```python
from build123d import *

# Parameters (mm, degrees)
SALIENTE_EXTRUIR1_DEPTH      = 22
CROQUIS2_W                   = 43.142135624
CROQUIS2_H                   = 44
SALIENTE_EXTRUIR2_DEPTH      = 8
CROQUIS3_W                   = 33.76116098
CROQUIS3_H                   = 8
CORTAR_EXTRUIR1_DEPTH        = 49.74935897
CROQUIS4_R                   = 11
SALIENTE_EXTRUIR4_DEPTH      = 2
CROQUIS7_R                   = 16
CROQUIS7_R_2                 = 2.6
SALIENTE_EXTRUIR5_DEPTH      = 2
CROQUIS6_W                   = 28
CROQUIS6_H                   = 12
CORTAR_EXTRUIR3_DEPTH        = 13
SALIENTE_EXTRUIR6_DEPTH      = 12
SALIENTE_EXTRUIR6_DEPTH_BACK = 3.8
CROQUIS8_W                   = 12
CROQUIS8_H                   = 12
CROQUIS8_R                   = 1.6
CROQUIS9_W                   = 2.5
CROQUIS9_H                   = 5.6
CORTAR_EXTRUIR4_DEPTH        = 10
CROQUIS11_W                  = 43.142135624
CROQUIS11_H                  = 46
SALIENTE_EXTRUIR8_DEPTH      = 30
CROQUIS12_W                  = 37.142135624
CROQUIS12_H                  = 28
CORTAR_EXTRUIR5_DEPTH        = 44
CROQUIS14_W                  = 13
CROQUIS14_H                  = 13
CORTAR_EXTRUIR7_DEPTH        = 25
CROQUIS13_R                  = 4.7625
CORTAR_EXTRUIR6_DEPTH        = 2
SALIENTE_EXTRUIR9_DEPTH      = 25
CROQUIS16_W                  = 13
CROQUIS16_H                  = 13
SALIENTE_EXTRUIR11_DEPTH     = 3.2


with BuildPart() as part:
    # Croquis1 → Saliente-Extruir1 (new, symmetric)
    with BuildSketch(Plane.XY):
        Polygon((26.5, -21.571067812), (26.5, 21.571067812), (21.571067812, 26.5), (-21.571067812, 26.5), (-26.5, 21.571067812), (-26.5, -21.571067812), (-21.571067812, -26.5), (21.571067812, -26.5), align=None)
        Polygon((-19.5, -21.5), (-21.5, -19.5), (-21.5, 19.5), (-19.5, 21.5), (19.5, 21.5), (21.5, 19.5), (21.5, -19.5), (19.5, -21.5), align=None, mode=Mode.SUBTRACT)
    extrude(amount=SALIENTE_EXTRUIR1_DEPTH, both=True)

    # Croquis2 → Saliente-Extruir2 (add)
    with BuildSketch(Plane.XZ.offset(26.5)):
        Rectangle(CROQUIS2_W, CROQUIS2_H)
    extrude(amount=SALIENTE_EXTRUIR2_DEPTH)

    # Croquis3 → Cortar-Extruir1 (cut, through all)
    with BuildSketch(Plane.XY):
        with Locations((0, -25.5)):
            Rectangle(CROQUIS3_W, CROQUIS3_H)
    extrude(amount=-CORTAR_EXTRUIR1_DEPTH, mode=Mode.SUBTRACT)

    # Croquis4 → Saliente-Extruir4 (add)
    with BuildSketch(Plane(origin=(0, 0, 22), x_dir=(-1, 0, 0), z_dir=(0, 0, -1))):
        Polygon((-26.5, -21.571067812), (-21.571067812, -26.5), (-21.571067812, -34.5), (21.571067812, -34.5), (21.571067812, -26.5), (26.5, -21.571067812), (26.5, 21.571067812), (21.571067812, 26.5), (-21.571067812, 26.5), (-26.5, 21.571067812), align=None)
        Circle(CROQUIS4_R, mode=Mode.SUBTRACT)
    extrude(amount=-SALIENTE_EXTRUIR4_DEPTH)

    # Croquis7 → Saliente-Extruir5 (add)
    with BuildSketch(Plane.XY.offset(24)):
        with Locations(Location((0, 0, 0), (0, 0, 180))):
            Circle(CROQUIS7_R)
        Circle(CROQUIS7_R_2, mode=Mode.SUBTRACT)
    extrude(amount=SALIENTE_EXTRUIR5_DEPTH)

    # Croquis6 → Cortar-Extruir3 (cut)
    with BuildSketch(Plane(origin=(0, -29.5, 0), x_dir=(1, 0, 0), z_dir=(0, 1, 0))):
        with Locations((0, 12)):
            Rectangle(CROQUIS6_W, CROQUIS6_H)
    extrude(amount=-CORTAR_EXTRUIR3_DEPTH, mode=Mode.SUBTRACT)

    # Croquis8 → Saliente-Extruir6 (add, two sides: drawn at the far end of the back side and taken through both)
    # profile 1 of 2: a face of its own
    with BuildSketch(Plane.XY.offset(-SALIENTE_EXTRUIR6_DEPTH_BACK)):
        with Locations((-32.5, -6)):
            Rectangle(CROQUIS8_W, CROQUIS8_H)
        with Locations((-32.5, -6)):
            Circle(CROQUIS8_R, mode=Mode.SUBTRACT)
    # profile 2 of 2: a face of its own
    with BuildSketch(Plane.XY.offset(-SALIENTE_EXTRUIR6_DEPTH_BACK)):
        with Locations((32.5, -6)):
            Rectangle(CROQUIS8_W, CROQUIS8_H)
        with Locations((32.5, -6)):
            Circle(CROQUIS8_R, mode=Mode.SUBTRACT)
    extrude(amount=SALIENTE_EXTRUIR6_DEPTH + SALIENTE_EXTRUIR6_DEPTH_BACK)

    # Croquis9 → Cortar-Extruir4 (cut)
    with BuildSketch(Plane(origin=(38.5, 0, 0), x_dir=(0, 0, -1), z_dir=(1, 0, 0))):
        with Locations((-4.1, -6)):
            Rectangle(CROQUIS9_W, CROQUIS9_H)
    cortar_extruir4 = extrude(amount=-CORTAR_EXTRUIR4_DEPTH, mode=Mode.SUBTRACT)

    # Simetría1: Cortar-Extruir4 across plane
    add(cortar_extruir4.mirror(Plane(origin=(0, 0, 0), x_dir=(0, 0, 1), z_dir=(1, 0, 0))), mode=Mode.SUBTRACT)

    # Croquis11 → Saliente-Extruir8 (add)
    with BuildSketch(Plane.XZ.offset(34.5)):
        with Locations((0, 1)):
            Rectangle(CROQUIS11_W, CROQUIS11_H)
    extrude(amount=SALIENTE_EXTRUIR8_DEPTH)

    # Croquis12 → Cortar-Extruir5 (cut)
    with BuildSketch(Plane(origin=(0, 0, -22), x_dir=(-1, 0, 0), z_dir=(0, 0, -1))):
        with Locations((0, -47.5)):
            Rectangle(CROQUIS12_W, CROQUIS12_H)
    extrude(amount=-CORTAR_EXTRUIR5_DEPTH, mode=Mode.SUBTRACT)

    # Croquis14 → Cortar-Extruir7 (cut)
    with BuildSketch(Plane.XY.offset(24)):
        with Locations((0, -35)):
            Rectangle(CROQUIS14_W, CROQUIS14_H)
    extrude(amount=-CORTAR_EXTRUIR7_DEPTH, mode=Mode.SUBTRACT)

    # Croquis13 → Cortar-Extruir6 (cut)
    with BuildSketch(Plane(origin=(0, 0, 22), x_dir=(-1, 0, 0), z_dir=(0, 0, -1))):
        with Locations((0, -47.5)):
            Circle(CROQUIS13_R)
    extrude(amount=-CORTAR_EXTRUIR6_DEPTH, mode=Mode.SUBTRACT)

    # Croquis15 → Saliente-Extruir9 (add)
    with BuildSketch(Plane(origin=(0, 0, 22), x_dir=(-1, 0, 0), z_dir=(0, 0, -1))):
        Polygon((-6.5, -33.5), (-18.571067812, -33.5), (-6.571067812, -45.5), (6.571067812, -45.5), (18.571067812, -33.5), (6.5, -33.5), (6.5, -41.5), (-6.5, -41.5), align=None)
    extrude(amount=SALIENTE_EXTRUIR9_DEPTH)

    # Croquis16 → Saliente-Extruir11 (add)
    with BuildSketch(Plane(origin=(0, 0, -3), x_dir=(-1, 0, 0), z_dir=(0, 0, -1))):
        with Locations((0, -35)):
            Rectangle(CROQUIS16_W, CROQUIS16_H)
    extrude(amount=-SALIENTE_EXTRUIR11_DEPTH)


solid = part.part
```
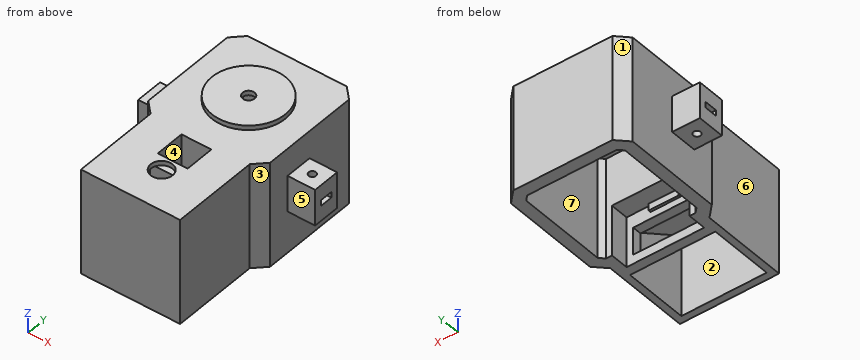
Read the model definition and answer for the solid it produces. Units are mm, in the model's axes. Face numbers are marked on the shaded views. A direction names the side the tool comes from. Coordinates: 2 decimals unless noted, no trailing zeros. Write each loop counter-clockwise with the first axis right and the second up, starting at its lowest first coordinate (ties: lowest second). Pieces come first, ordered by that corner, then holes. Notation, with made-up numbers: (89.25, 32) -> (119.25, 32) arc R35 cw to (119.25, 66) -> close; hole circle Ø2 at (11, 1.5). An arc over 180 degrees is marked (long way). Answer as a JSON object with one key per item and string values.
Q1. Determine the mould class of the marked faces 1, 2, 3 and 4 for opening direction Y: pulls with the +Y half, pulls with the -Y half, needs draft (parallel to the pull), parting line crosses it, or undercut.
The answers:
{"face 1": "pulls with the +Y half", "face 2": "undercut", "face 3": "pulls with the -Y half", "face 4": "undercut"}
Q2. The part is cut by section D-D on z = 16.5. Give the vertices of the cut face in (x, y), then the cut area to 3 significant figures.
The answers:
{"outline": "(-26.5, -21.57) -> (-21.57, -26.5) -> (-21.57, -64.5) -> (21.57, -64.5) -> (21.57, -26.5) -> (26.5, -21.57) -> (26.5, 21.57) -> (21.57, 26.5) -> (-21.57, 26.5) -> (-26.5, 21.57) -> close; hole (-21.5, -19.5) -> (-19.5, -21.5) -> (19.5, -21.5) -> (21.5, -19.5) -> (21.5, 19.5) -> (19.5, 21.5) -> (-19.5, 21.5) -> (-21.5, 19.5) -> close; hole (-18.57, -61.5) -> (18.57, -61.5) -> (18.57, -33.5) -> (6.57, -45.5) -> (-6.57, -45.5) -> (-18.57, -33.5) -> close; hole (-6.5, -41.5) -> (6.5, -41.5) -> (6.5, -28.5) -> (-6.5, -28.5) -> close", "area": "1,650 mm2"}
Q3. Flat-ended cylindrical pins translate along their axes: pin 1 Ø3.5 at (x, y) = (33, -6.5) entering from -Z; pin 2 Ø13 at (x, y) = (33.5, -3.5) entering from +Z; pin 3 Ø5 at (y, z) = (-15.5, -9) entering from +X. Find the tip coordinate at first contact, or state that the pin passes through.
The answers:
{"pin 1": "stops at z = -3.8", "pin 2": "stops at z = 12", "pin 3": "stops at x = 26.5"}
Q4. The part is cut by section A-A on x = 32.5. Give the vertices of the cut face in (y, z), then the cut area to 3 significant figures.
The answers:
{"outline": "(-12, -3.8) -> (-7.6, -3.8) -> (-7.6, 2.85) -> (-8.8, 2.85) -> (-8.8, 5.35) -> (-7.6, 5.35) -> (-7.6, 12) -> (-12, 12) -> close; (-4.4, -3.8) -> (0, -3.8) -> (0, 12) -> (-4.4, 12) -> (-4.4, 5.35) -> (-3.2, 5.35) -> (-3.2, 2.85) -> (-4.4, 2.85) -> close", "area": "133 mm2"}
Q5. A tool of negligible diameter and unlimited length cuts with its end or side. For the marked faces 5, 6 and 7, from which of +Z, -Z, +X, -X, +Y, -Y can it reach the whole face along a straight path? Write none if from no direction.
The answers:
{"face 5": "+Z, -Z, +X, -Y", "face 6": "+Z, -Z, -X, -Y", "face 7": "-Z"}
Q6. The part is cut by section B-B on y = -47.5. Give the vertices of the cut face in (x, z).
The answers:
{"outline": "(-21.57, -22) -> (-18.57, -22) -> (-18.57, 22) -> (-4.76, 22) -> (-4.76, 24) -> (-21.57, 24) -> close; (4.76, 22) -> (18.57, 22) -> (18.57, -22) -> (21.57, -22) -> (21.57, 24) -> (4.76, 24) -> close"}
Q7. Consider line 1 (X direction, y = -6, z = -0.25); line 2 (Y direction, x = 0, z = 22.8); line 3 (X direction, y = -5.5, z = 17.5). Determine where each line is inside the solid, lowest interval first. Write a range as [from, to].
The answers:
{"line 1": "x = [-38.5, -34.1], [-30.9, -21.5], [21.5, 30.9], [34.1, 38.5]", "line 2": "y = [-64.5, -52.26], [-42.74, -41.5], [-28.5, -11], [11, 26.5]", "line 3": "x = [-26.5, -21.5], [21.5, 26.5]"}
